```python
from build123d import *

# Parameters (mm, degrees)
BOSS_EXTRUDE1_DEPTH   = 15
BOSS_EXTRUDE1_2_DEPTH = 15
BOSS_EXTRUDE2_DEPTH   = 50
BOSS_EXTRUDE3_DEPTH   = 70
BOSS_EXTRUDE4_DEPTH   = 60
BOSS_EXTRUDE5_DEPTH   = 15


with BuildPart() as part:
    # Sketch1 → Boss-Extrude1 (new body)
    with BuildSketch(Plane(origin=(0, 0, 0), x_dir=(1, 0, 0), z_dir=(0, 1, 0))):
        with BuildLine():
            ThreePointArc((-31.622776602, -37.725821986), (-34.145257219, -30.413566094), (-35, -22.725821986))
            Line((-35, -22.725821986), (-35, 7.274178014))
            Line((-35, 7.274178014), (-40, 7.274178014))
            Line((-40, 7.274178014), (-40, 22.274178014))
            Line((-40, 22.274178014), (-60, 22.274178014))
            Line((-60, 22.274178014), (-60, 2.274178014))
            Line((-60, 2.274178014), (-50, -2.725821986))
            Line((-50, -2.725821986), (-50, -22.725821986))
            Line((-50, -22.725821986), (-60, -27.725821986))
            Line((-60, -27.725821986), (-60, -37.725821986))
            Line((-60, -37.725821986), (-31.622776602, -37.725821986))
        make_face()
    extrude(amount=BOSS_EXTRUDE1_DEPTH)



with BuildPart() as body_2:
    # Sketch1 → Boss-Extrude1 2 (new body)
    with BuildSketch(Plane(origin=(0, 0, 0), x_dir=(1, 0, 0), z_dir=(0, 1, 0))):
        with BuildLine():
            ThreePointArc((35, -22.725821986), (34.145257219, -30.413566094), (31.622776602, -37.725821986))
            Line((31.622776602, -37.725821986), (60, -37.725821986))
            Line((60, -37.725821986), (60, -27.725821986))
            Line((60, -27.725821986), (50, -22.725821986))
            Line((50, -22.725821986), (50, -2.725821986))
            Line((50, -2.725821986), (60, 2.274178014))
            Line((60, 2.274178014), (60, 22.274178014))
            Line((60, 22.274178014), (40, 22.274178014))
            Line((40, 22.274178014), (40, 7.274178014))
            Line((40, 7.274178014), (35, 7.274178014))
            Line((35, 7.274178014), (35, -22.725821986))
        make_face()
    extrude(amount=BOSS_EXTRUDE1_2_DEPTH)


with BuildPart() as part_1:
    add(part.part)

    add(body_2.part)  # Boss-Extrude2 merges body 2
    # Sketch1_3 → Boss-Extrude2 (add)
    with BuildSketch(Plane(origin=(0, 0, 0), x_dir=(1, 0, 0), z_dir=(0, 1, 0))):
        with BuildLine():
            Line((-22.912878475, -22.725821986), (-35, -22.725821986))
            ThreePointArc((-35, -22.725821986), (-34.145257219, -30.413566094), (-31.622776602, -37.725821986))
            ThreePointArc((-31.622776602, -37.725821986), (-18.708286934, -52.306220902), (0, -57.725821986))
            Line((0, -57.725821986), (0, -37.725821986))
            ThreePointArc((0, -37.725821986), (-13.693063938, -33.64232265), (-22.912878475, -22.725821986))
        make_face()
        with BuildLine():
            ThreePointArc((22.912878475, -22.725821986), (13.693063938, -33.64232265), (0, -37.725821986))
            Line((0, -37.725821986), (0, -57.725821986))
            ThreePointArc((0, -57.725821986), (18.708286934, -52.306220902), (31.622776602, -37.725821986))
            ThreePointArc((31.622776602, -37.725821986), (34.145257219, -30.413566094), (35, -22.725821986))
            Line((35, -22.725821986), (22.912878475, -22.725821986))
        make_face()
    extrude(amount=BOSS_EXTRUDE2_DEPTH)

    # Sketch1_4 → Boss-Extrude3 (add)
    with BuildSketch(Plane(origin=(0, 0, 0), x_dir=(1, 0, 0), z_dir=(0, 1, 0))):
        with BuildLine():
            Line((-35, 7.274178014), (-35, -22.725821986))
            Line((-35, -22.725821986), (-22.912878475, -22.725821986))
            ThreePointArc((-22.912878475, -22.725821986), (-24.540895298, -7.956706975), (-17.5, 5.127749085))
            Line((-17.5, 5.127749085), (-17.5, 22.274178014))
            Line((-17.5, 22.274178014), (-35, 22.274178014))
            Line((-35, 22.274178014), (-40, 22.274178014))
            Line((-40, 22.274178014), (-40, 7.274178014))
            Line((-40, 7.274178014), (-35, 7.274178014))
        make_face()
        with BuildLine():
            ThreePointArc((25, -12.725821986), (24.472657823, -17.833563079), (22.912878475, -22.725821986))
            Line((22.912878475, -22.725821986), (35, -22.725821986))
            Line((35, -22.725821986), (35, 7.274178014))
            Line((35, 7.274178014), (40, 7.274178014))
            Line((40, 7.274178014), (40, 22.274178014))
            Line((40, 22.274178014), (35, 22.274178014))
            Line((35, 22.274178014), (17.5, 22.274178014))
            Line((17.5, 22.274178014), (17.5, 5.127749085))
            ThreePointArc((17.5, 5.127749085), (23.048861143, -3.043363621), (25, -12.725821986))
        make_face()
    extrude(amount=BOSS_EXTRUDE3_DEPTH)

    # Sketch1_5 → Boss-Extrude4 (add)
    with BuildSketch(Plane(origin=(0, 0, 0), x_dir=(1, 0, 0), z_dir=(0, 1, 0))):
        with BuildLine():
            Line((-17.5, 22.274178014), (-17.5, 5.127749085))
            ThreePointArc((-17.5, 5.127749085), (-9.451474044, 10.418715995), (0, 12.274178014))
            Line((0, 12.274178014), (0, 22.274178014))
            Line((0, 22.274178014), (-17.5, 22.274178014))
        make_face()
        with BuildLine():
            Line((0, 22.274178014), (0, 12.274178014))
            ThreePointArc((0, 12.274178014), (9.451474044, 10.418715995), (17.5, 5.127749085))
            Line((17.5, 5.127749085), (17.5, 22.274178014))
            Line((17.5, 22.274178014), (0, 22.274178014))
        make_face()
    extrude(amount=BOSS_EXTRUDE4_DEPTH)

    # Sketch3 → Boss-Extrude5 (add)
    with BuildSketch(Plane(origin=(0, 0, -22.274178014), x_dir=(-1, 0, 0), z_dir=(0, 0, -1))):
        Polygon((60, 15), (40, 15), (40, 70), align=None)
        Polygon((-60, 15), (-40, 15), (-40, 70), align=None)
    extrude(amount=-BOSS_EXTRUDE5_DEPTH)


solid = part_1.part
```
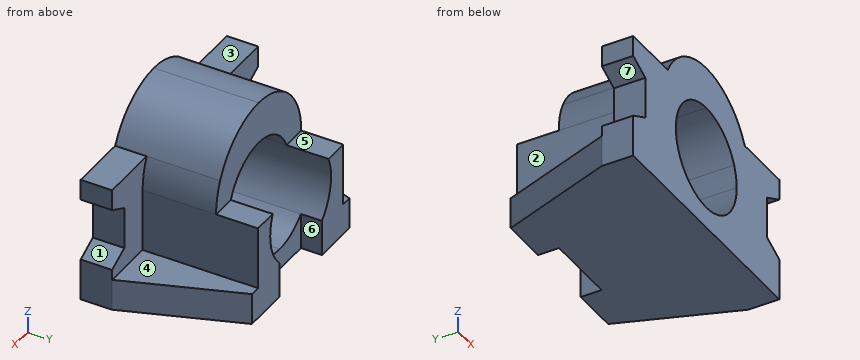
Here's how the part is built. I have some questions about the finished solid (model axes, mm). Face numbers are marked on the shaded views. A direction names the side the tool comes from. Give positions to 0.01 mm unless a question says otherwise; leave off trailing zeros. Write each loop counter-clockwise with the first axis right and the second up, starting at its lowest first coordinate (ties: lowest second). Pieces come first, ordered by that corner, then holes.
(1) Will these pins go through, and if not, where does the flat tip stop? pin 1 (10 mm diameter, centred on x = -21.5, y = 10, fed in from +Z); pin 2 (3 mm diameter, centred on y = 64.5, z = -16.5, fed in from -X); pin 3 (7.5 mm diameter, centred on x = 49.5, y = 31.5, fed in from +Z); pin 4 (2 mm diameter, centred on x = 17.5, z = 30, fed in from -Y).
Output values:
pin 1: stops at z = 53.59
pin 2: stops at x = -42.55
pin 3: stops at z = -7.27
pin 4: stops at y = 0
(2) On a 3-axis mill with a long thin cutter (end or side, diameter ignored), from which of +Z, -Z, +X, -X, +Y, -Y can I reach the whole of each face in a straight line? I mean the marked faces 1, 2, 3 and 4. Say none if no direction works.
Output values:
face 1: +X, +Y, -Y
face 2: +Z, -X, +Y
face 3: +Z, -X, +Y, -Y
face 4: +Z, +X, +Y
(3) Imagine slicing it at D-D, the plane y = 62.5. Write out the boundary of the cut face in (x, z), and give its area (3 significant figures).
Output values:
outline: (-42.73, -22.27) - (-17.5, -22.27) - (-17.5, -5.13) arc R25 cw to (-22.91, 22.73) - (-35, 22.73) - (-35, -7.27) - (-42.73, -7.27) - close; (17.5, -22.27) - (42.73, -22.27) - (42.73, -7.27) - (35, -7.27) - (35, 22.73) - (22.91, 22.73) arc R25 cw to (17.5, -5.13) - close
area: 1,490 mm2
(4) Imagine slicing it at C-C, the plane z = 35.5. Write out the boundary of the cut face in (x, y), and give its area (3 significant figures).
Output values:
outline: (-60, 0) - (-10.31, 0) - (-10.31, 50) - (-32.59, 50) - (-32.59, 15) - (-60, 15) - close; (10.31, 0) - (60, 0) - (60, 15) - (32.59, 15) - (32.59, 50) - (10.31, 50) - close
area: 3,050 mm2
(5) Thinking about a two-plate mould opening in X: for the marked faces 5, 6 and 7, which applies, pulls with the +X half, pulls with the -X half, needs draft (parallel to the pull), parting line crosses it, or undercut?
Output values:
face 5: needs draft
face 6: undercut
face 7: pulls with the -X half
(6) Imagine slicing it at B-B, the plane x = 9. Write out the boundary of the cut face in (y, z).
Output values:
outline: (0, -22.27) - (60, -22.27) - (60, -10.6) - (0, -10.6) - close; (0, 36.05) - (50, 36.05) - (50, 56.55) - (0, 56.55) - close
(7) Imagine slicing it at A-A, the plane y = 37. Write out the boundary of the cut face in (x, z), and give its area (3 significant figures).
Output values:
outline: (-52, -22.27) - (52, -22.27) - (52, -7.27) - (35, -7.27) - (35, 22.73) arc R35 ccw to (-35, 22.73) - (-35, -7.27) - (-52, -7.27) - close; hole circle Ø50 at (0, 12.73)
area: 3,620 mm2
(8) If I drill on L1, parallel to Y at x = -46, z = 15.5; L2, parallel to Z at x = -38, y = 28.5; L3, parallel to X at y = 14.5, z = -3.5, over which ranges is the centre line in solid material (lowest first)?
Output values:
L1: y = 0 to 15
L2: z = -22.27 to -7.27
L3: x = -60 to -19.02, 19.02 to 60
